CAD build for the part. Positions are in the model's coordinates, mm. Give positions to 0.01 mm unless a question says otherwise; leave off trailing zeros. Write each loop counter-clockwise with the first axis right and the second up, starting at its lowest first coordinate (ties: lowest second). Pieces come first, ordered by that corner, then holes. Notation, with made-up numbers: (58.25, -28) - (109.25, -28) arc R31 ccw to (109.25, 2) - close; hole circle Ø2 at (27.5, -30.5). An arc over 180 degrees is marked (long way). Answer as a JSON object with one key per item and string values.
from build123d import *

# Parameters (mm, degrees)
SKETCH_1_R             = 42
SM_BASE_FLANGE_1_DEPTH = 2
CUT_EXTRUDE_1_REACH    = 61.431
SKETCH_6_R             = 2.1
SKETCH_6_R_2           = 3
SKETCH_6_R_3           = 2
SKETCH_6_W             = 8
SKETCH_6_H             = 5
SKETCH_6_W_2           = 5
SKETCH_6_H_2           = 8
FILLET_1_R             = 1


# Sheet-metal steps are written as plain solids
with BuildPart() as part:
    # Sketch 1 → 基体-法兰1 (new body)
    with BuildSketch(Plane(origin=(0, 0, 0), x_dir=(1, 0, 0), z_dir=(0, 1, 0))):
        with Locations(Location((0, 0, 0), (0, 0, 270))):
            Circle(SKETCH_1_R)
    extrude(amount=-SM_BASE_FLANGE_1_DEPTH)

    # 草图6 → 切除-拉伸1 (cut, up to next)
    with BuildSketch(Plane(origin=(0, 0, 0), x_dir=(1, 0, 0), z_dir=(0, 1, 0)), mode=Mode.PRIVATE) as cut_extrude_1_sk1:
        with Locations(Location((0, 35, 0), (0, 0, 270))):
            Circle(SKETCH_6_R)
    cut_extrude_1_tool1 = extrude(cut_extrude_1_sk1.sketch, amount=-CUT_EXTRUDE_1_REACH, mode=Mode.PRIVATE) & part.part
    # 草图6 → 切除-拉伸1 (cut, up to next)
    with BuildSketch(Plane(origin=(0, 0, 0), x_dir=(1, 0, 0), z_dir=(0, 1, 0)), mode=Mode.PRIVATE) as cut_extrude_1_sk2:
        with Locations(Location((35, 0, 0), (0, 0, 270))):
            Circle(SKETCH_6_R)
    cut_extrude_1_tool2 = extrude(cut_extrude_1_sk2.sketch, amount=-CUT_EXTRUDE_1_REACH, mode=Mode.PRIVATE) & part.part
    # 草图6 → 切除-拉伸1 (cut, up to next)
    with BuildSketch(Plane(origin=(0, 0, 0), x_dir=(1, 0, 0), z_dir=(0, 1, 0)), mode=Mode.PRIVATE) as cut_extrude_1_sk3:
        with Locations(Location((0, -35, 0), (0, 0, 270))):
            Circle(SKETCH_6_R)
    cut_extrude_1_tool3 = extrude(cut_extrude_1_sk3.sketch, amount=-CUT_EXTRUDE_1_REACH, mode=Mode.PRIVATE) & part.part
    # 草图6 → 切除-拉伸1 (cut, up to next)
    with BuildSketch(Plane(origin=(0, 0, 0), x_dir=(1, 0, 0), z_dir=(0, 1, 0)), mode=Mode.PRIVATE) as cut_extrude_1_sk4:
        with Locations(Location((-35, 0, 0), (0, 0, 270))):
            Circle(SKETCH_6_R)
    cut_extrude_1_tool4 = extrude(cut_extrude_1_sk4.sketch, amount=-CUT_EXTRUDE_1_REACH, mode=Mode.PRIVATE) & part.part
    # 草图6 → 切除-拉伸1 (cut, up to next)
    with BuildSketch(Plane(origin=(0, 0, 0), x_dir=(1, 0, 0), z_dir=(0, 1, 0)), mode=Mode.PRIVATE) as cut_extrude_1_sk5:
        with Locations(Location((0, 0, 0), (0, 0, 270))):
            Circle(SKETCH_6_R_2)
    cut_extrude_1_tool5 = extrude(cut_extrude_1_sk5.sketch, amount=-CUT_EXTRUDE_1_REACH, mode=Mode.PRIVATE) & part.part
    # 草图6 → 切除-拉伸1 (cut, up to next)
    with BuildSketch(Plane(origin=(0, 0, 0), x_dir=(1, 0, 0), z_dir=(0, 1, 0)), mode=Mode.PRIVATE) as cut_extrude_1_sk6:
        with Locations(Location((-5, 5, 0), (0, 0, 270))):
            Circle(SKETCH_6_R_3)
    cut_extrude_1_tool6 = extrude(cut_extrude_1_sk6.sketch, amount=-CUT_EXTRUDE_1_REACH, mode=Mode.PRIVATE) & part.part
    # 草图6 → 切除-拉伸1 (cut, up to next)
    with BuildSketch(Plane(origin=(0, 0, 0), x_dir=(1, 0, 0), z_dir=(0, 1, 0)), mode=Mode.PRIVATE) as cut_extrude_1_sk7:
        with Locations(Location((5, 5, 0), (0, 0, 270))):
            Circle(SKETCH_6_R_3)
    cut_extrude_1_tool7 = extrude(cut_extrude_1_sk7.sketch, amount=-CUT_EXTRUDE_1_REACH, mode=Mode.PRIVATE) & part.part
    # 草图6 → 切除-拉伸1 (cut, up to next)
    with BuildSketch(Plane(origin=(0, 0, 0), x_dir=(1, 0, 0), z_dir=(0, 1, 0)), mode=Mode.PRIVATE) as cut_extrude_1_sk8:
        with Locations(Location((5, -5, 0), (0, 0, 270))):
            Circle(SKETCH_6_R_3)
    cut_extrude_1_tool8 = extrude(cut_extrude_1_sk8.sketch, amount=-CUT_EXTRUDE_1_REACH, mode=Mode.PRIVATE) & part.part
    # 草图6 → 切除-拉伸1 (cut, up to next)
    with BuildSketch(Plane(origin=(0, 0, 0), x_dir=(1, 0, 0), z_dir=(0, 1, 0)), mode=Mode.PRIVATE) as cut_extrude_1_sk9:
        with Locations(Location((-5, -5, 0), (0, 0, 270))):
            Circle(SKETCH_6_R_3)
    cut_extrude_1_tool9 = extrude(cut_extrude_1_sk9.sketch, amount=-CUT_EXTRUDE_1_REACH, mode=Mode.PRIVATE) & part.part
    # 草图6 → 切除-拉伸1 (cut, up to next)
    with BuildSketch(Plane(origin=(0, 0, 0), x_dir=(1, 0, 0), z_dir=(0, 1, 0)), mode=Mode.PRIVATE) as cut_extrude_1_sk10:
        with Locations((0, 25)):
            Rectangle(SKETCH_6_W, SKETCH_6_H)
    cut_extrude_1_tool10 = extrude(cut_extrude_1_sk10.sketch, amount=-CUT_EXTRUDE_1_REACH, mode=Mode.PRIVATE) & part.part
    # 草图6 → 切除-拉伸1 (cut, up to next)
    with BuildSketch(Plane(origin=(0, 0, 0), x_dir=(1, 0, 0), z_dir=(0, 1, 0)), mode=Mode.PRIVATE) as cut_extrude_1_sk11:
        with Locations((15, 0)):
            Rectangle(SKETCH_6_W_2, SKETCH_6_H_2)
    cut_extrude_1_tool11 = extrude(cut_extrude_1_sk11.sketch, amount=-CUT_EXTRUDE_1_REACH, mode=Mode.PRIVATE) & part.part
    # 草图6 → 切除-拉伸1 (cut, up to next)
    with BuildSketch(Plane(origin=(0, 0, 0), x_dir=(1, 0, 0), z_dir=(0, 1, 0)), mode=Mode.PRIVATE) as cut_extrude_1_sk12:
        with Locations((-15, 0)):
            Rectangle(SKETCH_6_W_2, SKETCH_6_H_2)
    cut_extrude_1_tool12 = extrude(cut_extrude_1_sk12.sketch, amount=-CUT_EXTRUDE_1_REACH, mode=Mode.PRIVATE) & part.part
    add(cut_extrude_1_tool1.solids().sort_by_distance((0, 0, -35))[0], mode=Mode.SUBTRACT)
    add(cut_extrude_1_tool2.solids().sort_by_distance((35, 0, 0))[0], mode=Mode.SUBTRACT)
    add(cut_extrude_1_tool3.solids().sort_by_distance((0, 0, 35))[0], mode=Mode.SUBTRACT)
    add(cut_extrude_1_tool4.solids().sort_by_distance((-35, 0, 0))[0], mode=Mode.SUBTRACT)
    add(cut_extrude_1_tool5.solids().sort_by_distance((0, 0, 0))[0], mode=Mode.SUBTRACT)
    add(cut_extrude_1_tool6.solids().sort_by_distance((-5, 0, -5))[0], mode=Mode.SUBTRACT)
    add(cut_extrude_1_tool7.solids().sort_by_distance((5, 0, -5))[0], mode=Mode.SUBTRACT)
    add(cut_extrude_1_tool8.solids().sort_by_distance((5, 0, 5))[0], mode=Mode.SUBTRACT)
    add(cut_extrude_1_tool9.solids().sort_by_distance((-5, 0, 5))[0], mode=Mode.SUBTRACT)
    add(cut_extrude_1_tool10.solids().sort_by_distance((0, 0, -25))[0], mode=Mode.SUBTRACT)
    add(cut_extrude_1_tool11.solids().sort_by_distance((15, 0, 0))[0], mode=Mode.SUBTRACT)
    add(cut_extrude_1_tool12.solids().sort_by_distance((-15, 0, 0))[0], mode=Mode.SUBTRACT)

    # 圆角1
    fillet_1_edges = [part.edges().sort_by_distance(p)[0] for p in [
        (17.5, -1, -4),
        (17.5, -1, 4),
        (12.5, -1, 4),
        (12.5, -1, -4),
        (-12.5, -1, -4),
        (-12.5, -1, 4),
        (-17.5, -1, 4),
        (-17.5, -1, -4),
        (-4, -1, -22.5),
        (-4, -1, -27.5),
        (4, -1, -27.5),
        (4, -1, -22.5),
    ]]
    fillet(fillet_1_edges, radius=FILLET_1_R)


solid = part.part
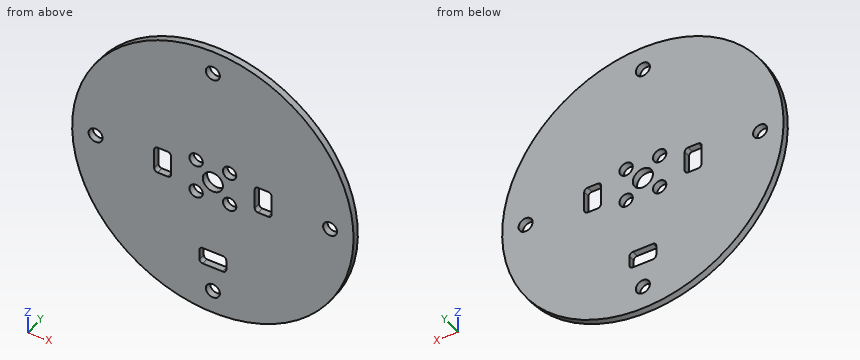
Item 1: Cut at C-C (x = -35). Give the cut face in (y, z).
Entries:
{"outline": "(-2, -23.22) - (0, -23.22) - (0, -2.1) - (-2, -2.1) - close; (-2, 2.1) - (0, 2.1) - (0, 23.22) - (-2, 23.22) - close"}
Item 2: Probe line 1 (X direction, y = -1.5, z = 0); line 2 (X direction, y = -0.7, z = 5); line 3 (X direction, y = -0.1, z = -0.5). List the from-to ranges inside material, lowest first. Write a range as from..to.
Entries:
{"line 1": "-42..-37.1, -32.9..-17.5, -12.5..-3, 3..12.5, 17.5..32.9, 37.1..42", "line 2": "-41.7..-7, -3..3, 7..41.7", "line 3": "-42..-37.04, -32.96..-17.5, -12.5..-2.96, 2.96..12.5, 17.5..32.96, 37.04..42"}
Item 3: Flat gauge pins, fed straight in: P1, Ø1, axis at x = -15, y = -0.5, coming from the -Z side; P2, Ø2.5, axis at x = 35, z = 0, coming from the -Y side; P3, Ø0.6, axis at x = -15.5, y = -1.5, coming from the +Z side; P4, Ø5, axis at x = -5, z = -5, coming from the -Y side. Where does each tip first touch, or does it go through?
Entries:
{"P1": "z = -39.42", "P2": "through", "P3": "z = 39.15", "P4": "y = -2"}
Item 4: Cut at D-D (y = -1.05). State how many separate pieces and enclosed holes the cut face has, and give its area (3 significant figures).
Entries:
{"separate pieces": "1", "enclosed holes": "12", "area": "5,290 mm2"}
Item 5: Cut at B-B (x = 5). Give the cut face in (y, z), and give its area (3 significant figures).
Entries:
{"outline": "(-2, -41.7) - (0, -41.7) - (0, -7) - (-2, -7) - close; (-2, -3) - (0, -3) - (0, 3) - (-2, 3) - close; (-2, 7) - (0, 7) - (0, 41.7) - (-2, 41.7) - close", "area": "151 mm2"}
Item 6: Cut at A-A (z = 0). Give the cut face in (x, y), and give its area (3 significant figures).
Entries:
{"outline": "(-42, -2) - (-37.1, -2) - (-37.1, 0) - (-42, 0) - close; (-32.9, -2) - (-17.5, -2) - (-17.5, 0) - (-32.9, 0) - close; (-12.5, -2) - (-3, -2) - (-3, 0) - (-12.5, 0) - close; (3, -2) - (12.5, -2) - (12.5, 0) - (3, 0) - close; (17.5, -2) - (32.9, -2) - (32.9, 0) - (17.5, 0) - close; (37.1, -2) - (42, -2) - (42, 0) - (37.1, 0) - close", "area": "119 mm2"}
